Design review of the part built by this model. Coordinates are the model's own, in mm. A direction names the side the tool comes from. Give positions to 0.01 mm unless a question says otherwise; leave off trailing zeros. Order: outer loops, then holes, each group sorted by start corner. A loop starts at its lowest first (then second) coordinate and runs counter-clockwise, first axis right, second up. Notation, with made-up numbers: M -31.75,34.25 L -26.75,34.25 A19 cw -26.75,48.25 Z; hole C -40,15 d5. An arc over 180 degrees is marked long. Answer as a JSON object with one key per item and string values.
from build123d import *

# Parameters (mm, degrees)
F0_W     = 62
F0_H     = 32
F1_DEPTH = 14
F2_T     = -2.4


with BuildPart() as f1:
    # F0 (on Front) → F1 (new body)
    with BuildSketch(Plane.XZ):
        Rectangle(F0_W, F0_H)
    extrude(amount=F1_DEPTH)

    # F2
    f2_openings = [f1.faces().sort_by_distance(p)[0] for p in [
        (31, -7, 0),
        (-31, -7, 0),
    ]]
    offset(amount=F2_T, openings=f2_openings)


solid = f1.part
(1) We need section B-B (y = -9.5). Write out the cut boundary in (x, z), plus the area to 3 significant figures.
Checked values:
{"outline": "M -31,-16 L 31,-16 L 31,-13.6 L -31,-13.6 Z; M -31,13.6 L 31,13.6 L 31,16 L -31,16 Z", "area": "298 mm^2"}
(2) We need section C-C (x = 18.5). Write out the cut boundary in (y, z).
Checked values:
{"outline": "M -14,-16 L 0,-16 L 0,16 L -14,16 Z; hole M -11.6,-13.6 L -2.4,-13.6 L -2.4,13.6 L -11.6,13.6 Z"}
(3) Draft analysis for pull direction Z (two halves, no side actions). For faces 3 (the flat face through (0, 0, 0)), 4 (the flat face through (0, -2.4, 0)), 5 (the flat face through (0, -7, 16)), 6 (the flat face through (0, -7, -16)), state which applies: +Z half, -Z half, draft (parallel to the pull), parting line (faces both ways), or undercut.
Checked values:
{"face 3": "draft", "face 4": "undercut", "face 5": "+Z half", "face 6": "-Z half"}
(4) We need section A-A (z = 11). Write out the cut boundary in (x, y).
Checked values:
{"outline": "M -31,-14 L 31,-14 L 31,-11.6 L -31,-11.6 Z; M -31,-2.4 L 31,-2.4 L 31,0 L -31,0 Z"}
(5) To check wall thickness, follow L1, parallel to Z at x = 4, y = -10.25; L2, parallel to Y at x = -18, z = 9. State the ranges of each line that lie inside material, in increasing order. Write a range as from..to.
Checked values:
{"L1": "z = -16..-13.6, 13.6..16", "L2": "y = -14..-11.6, -2.4..0"}
(6) Tool access review of faces 1 (the flat face through (0, -14, 0)), 2 (the flat face through (0, -7, 13.6)): name each direction out of +Z, -Z, +X, -X, +Y, -Y from which nothing blocks a thin tool from reaching the whole face with its end or side.
Checked values:
{"face 1": "+Z, -Z, +X, -X, -Y", "face 2": "+X, -X"}
(7) Insertion check: pin 1 (3 mm diameter, centred on x = -9.5, z = -7, fed in from +Y); pin 2 (1 mm diameter, centred on y = -3.5, z = -8.5, fed in from +X). Each pin has a flat end and moves straight along its axis. Give the tip position at first contact, or say it passes through.
Checked values:
{"pin 1": "stops at y = 0", "pin 2": "passes through"}
